Design review of the part shown in the three views and the two pictorial views. Dimensions are in mm from the part's minimum x, y and z. A direction names the side the tool comes from. Coordinates: 2 decimals unless noted, no trailing zeros. Loops run counter-clockwise (first coordinate to the right, second up) from the corner with the lowest first, then second, coordinate; pieces in that order, holes last.
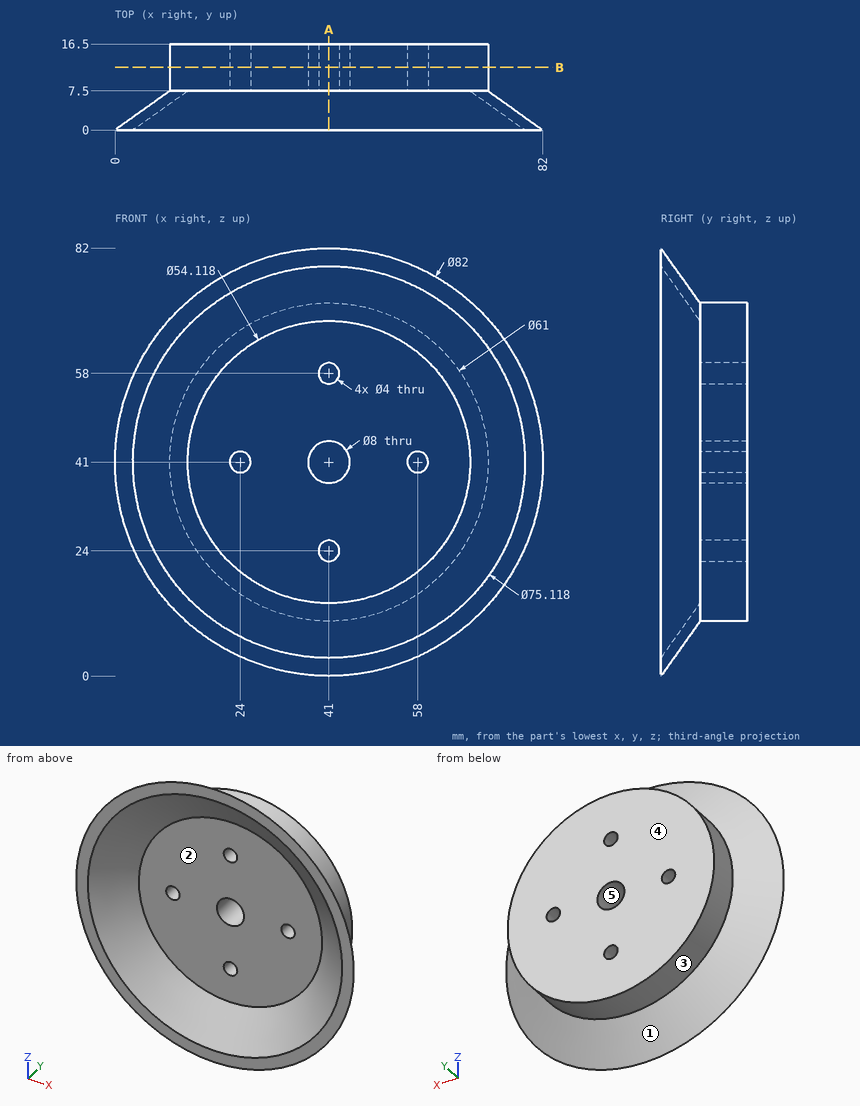
Q1. Consider section B-B (y = 12). State the section outline as (x, z) points.
Q2. For pin 1 Ø3 at (x, z) = (58, 41) entering from -Y; pin 2 Ø3 at (x, z) = (31, 59.5) entering from -Y; pin 3 Ø3 at (x, z) = (30, 72) entering from -Y; pin 4 Ø2 at (x, y) = (16, 5) entering from -Z (1 decimal), all flat-tipped, find the tip position at first contact; note any pin that passes through.
Q3. Wall thickness on probe 1 along X at (y, z) = (13, 41); probe 2 along Y at (x, z) = (46, 29); probe 3 along Z at (x, y) = (56.5, 5): over which ranges is each line inside the solid? List them lowest first.
Q4. The part is to be moulded in two halves that separate along Z. For the marked faces 3, 4 and 5, say which applies: +Z half, -Z half, draft (parallel to the pull), parting line (faces both ways), or undercut.
Q5. Machinability: for the marked faces 1 and 2, which of the approach directions +Z, -Z, +X, -X, +Y, -Y give a long, thin tool a straight path to every point of the face, cutting with its end or side? Answer none if there is none.
Q6. Consider section A-A (x = 41). State the section outline as (y, z) points.
Model answer:
1. outline: circle Ø61 at (41, 41); hole circle Ø4 at (24, 41); hole circle Ø8 at (41, 41); hole circle Ø4 at (41, 24); hole circle Ø4 at (41, 58); hole circle Ø4 at (58, 41)
2. pin 1: passes through
2. pin 2: stops at y = 7.5
2. pin 3: stops at y = 2.26
2. pin 4: stops at z = 15.7
3. probe 1: x = 10.5 to 22, 26 to 37, 45 to 56, 60 to 71.5
3. probe 2: y = 7.5 to 16.5
3. probe 3: z = 10.74 to 14.66, 67.34 to 71.26
4. face 3: parting line
4. face 4: draft
4. face 5: undercut
5. face 1: +Y
5. face 2: -Y
6. outline: (0, 0) - (7.5, 10.5) - (16.5, 10.5) - (16.5, 22) - (7.5, 22) - (7.5, 13.94) - (0, 3.44) - close; (0, 78.56) - (7.5, 68.06) - (7.5, 60) - (16.5, 60) - (16.5, 71.5) - (7.5, 71.5) - (0, 82) - close; (7.5, 26) - (16.5, 26) - (16.5, 37) - (7.5, 37) - close; (7.5, 45) - (16.5, 45) - (16.5, 56) - (7.5, 56) - close
